from build123d import *

# Parameters (mm, degrees)
F0_W     = 620
F0_H     = 250
F1_DEPTH = 12
F2_W     = 12
F2_H     = 250
F3_DEPTH = 300
F4_R     = 5


with BuildPart() as f1:
    # F0 (on Top) → F1 (new body)
    with BuildSketch(Plane.XY):
        with Locations((310, -125)):
            Rectangle(F0_W, F0_H)
    extrude(amount=-F1_DEPTH)

    # F2 (on Top) → F3 (join)
    with BuildSketch(Plane.XY):
        with Locations((-6, -125)):
            Rectangle(F2_W, F2_H)
        with Locations((626, -125)):
            Rectangle(F2_W, F2_H)
    extrude(amount=-F3_DEPTH)

    # F4
    f4_edges = [f1.edges().sort_by_distance(p)[0] for p in [
        (-12, -125, 0),
        (310, -250, 0),
        (632, -125, 0),
        (310, 0, 0),
    ]]
    fillet(f4_edges, radius=F4_R)


solid = f1.part
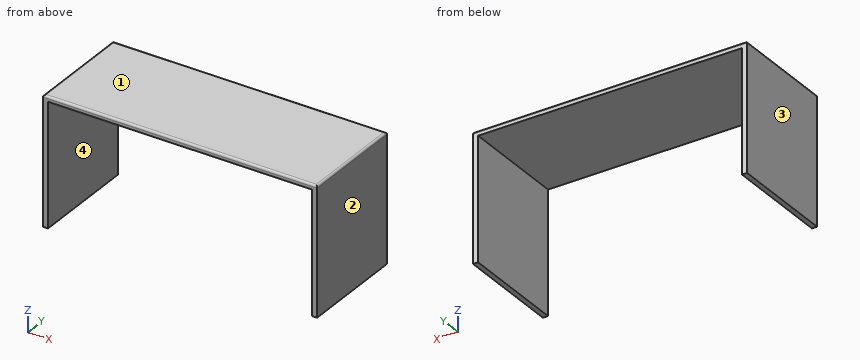
Source: CAD feature listing. Evaluate the final solid. Frame: model axes, mm. Face numbers are marked on the shaded views. Give positions to 0.01 mm unless a question says otherwise; leave off trailing zeros. Write each loop counter-clockwise with the first axis right and the second up, starting at its lowest first coordinate (ties: lowest second). Pieces come first, ordered by that corner, then holes. Notation, with made-up numbers: M 87.5,80 L 104.5,80 A26 ccw 104.5,101 Z; hole C 1,-1.75 d4. An arc over 180 degrees is marked long. Return JSON: item names as keys, results as strings. Group by question number.
1) Pin query (flat end, axial travel): P1, Ø2, axis at x = 427, y = -220.5, coming from the -Z side. Return the tip coordinate at first contact, or that it passes through.
2) Material intervals for line 1 along X through (y, z) = (-75, -101); line 2 along Z through (x, y) = (126, -145), sorted ascending. Write a range as [from, to].
3) Cut plane B-B, the plane y = -154. Output: boundary loops of the cut face in (x, z), plus the area to 3 significant figures.
4) Pull-direction query (X, two-part tool) for the marked faces 1, 2, 3 and 4; classes: pulls with the +X half, pulls with the -X half, needs draft (parallel to the pull), parting line crosses it, or undercut.
5) Cut plane A-A, the plane z = -64. Output: boundary loops of the cut face in (x, y), plus the area to 3 significant figures.
6) Cut plane C-C, the plane x = 349. Output: boundary loops of the cut face in (y, z).
Recorded:
{
 "1": {"P1": "stops at z = -12"},
 "2": {"line 1": "x = [-12, 0], [620, 632]", "line 2": "z = [-12, 0]"},
 "3": {"outline": "M -12,-300 L 0,-300 L 0,-12 L 620,-12 L 620,-300 L 632,-300 L 632,-5 A5 ccw 627,0 L -7,0 A5 ccw -12,-5 Z", "area": "14,600 mm²"},
 "4": {"face 1": "needs draft", "face 2": "pulls with the +X half", "face 3": "pulls with the -X half", "face 4": "undercut"},
 "5": {"outline": "M -12,-250 L 0,-250 L 0,0 L -12,0 Z; M 620,-250 L 632,-250 L 632,0 L 620,0 Z", "area": "6,000 mm²"},
 "6": {"outline": "M -250,-12 L 0,-12 L 0,-5 A5 ccw -5,0 L -245,0 A5 ccw -250,-5 Z"}
}
